Source: CAD feature listing. Evaluate the final solid. Frame: model axes, mm. A direction names the side the tool comes from. Give positions to 0.01 mm unless a question says otherwise; leave off trailing zeros. Order: outer loops, then holes, each group sorted by start corner. A loop starts at its lowest first (then second) coordinate and runs counter-clockwise, first axis right, second up.
```python
from build123d import *

# Parameters (mm, degrees)
SKETCH1_W           = 165
SKETCH1_H           = 137
BOSS_EXTRUDE1_DEPTH = 22
CUT_EXTRUDE1_DEPTH  = 165
FILLET1_R           = 3
SKETCH3_R           = 2.75
SKETCH3_R_2         = 1.45
CUT_EXTRUDE2_DEPTH  = 5
FILLET2_R           = 3
FILLET3_R           = 3


with BuildPart() as part:
    # Sketch1 → Boss-Extrude1 (new body)
    with BuildSketch(Plane(origin=(0, 0, 0), x_dir=(0, 0, -1), z_dir=(1, 0, 0))):
        Rectangle(SKETCH1_W, SKETCH1_H)
    extrude(amount=BOSS_EXTRUDE1_DEPTH)

    # Sketch2 → Cut-Extrude1 (cut)
    with BuildSketch(Plane.XY.offset(82.5)):
        Polygon((0, 48.5), (5, 48.5), (5, 53.5), (17, 53.5), (17, -53.5), (5, -53.5), (5, -43.5), (0, -43.5), align=None)
    extrude(amount=-CUT_EXTRUDE1_DEPTH, mode=Mode.SUBTRACT)

    # Fillet1
    fillet1_edges = [part.edges().sort_by_distance(p)[0] for p in [
        (22, -68.5, 0),
        (0, -43.5, 0),
        (0, 48.5, 0),
        (0, -68.5, 0),
        (0, 68.5, 0),
        (22, 68.5, 0),
    ]]
    fillet(fillet1_edges, radius=FILLET1_R)

    # Sketch3 → Cut-Extrude2 (cut)
    with BuildSketch(Plane.ZY.offset(-17)):
        with Locations(Location((0, -0.084265268, 0), (0, 0, 270))):
            Circle(SKETCH3_R)
        with Locations(Location((6.905, -0.084265268, 0), (0, 0, 270))):
            Circle(SKETCH3_R_2)
        with Locations(Location((4.882572324, -4.966837592, 0), (0, 0, 270))):
            Circle(SKETCH3_R_2)
        with Locations(Location((0, -6.989265268, 0), (0, 0, 270))):
            Circle(SKETCH3_R_2)
        with Locations(Location((-4.882572324, -4.966837592, 0), (0, 0, 270))):
            Circle(SKETCH3_R_2)
        with Locations(Location((-6.905, -0.084265268, 0), (0, 0, 270))):
            Circle(SKETCH3_R_2)
        with Locations(Location((-4.882572324, 4.798307056, 0), (0, 0, 270))):
            Circle(SKETCH3_R_2)
        with Locations(Location((0, 6.820734732, 0), (0, 0, 270))):
            Circle(SKETCH3_R_2)
        with Locations(Location((4.882572324, 4.798307056, 0), (0, 0, 270))):
            Circle(SKETCH3_R_2)
    extrude(amount=-CUT_EXTRUDE2_DEPTH, mode=Mode.SUBTRACT)

    # Fillet2
    fillet2_edges = [part.edges().sort_by_distance(p)[0] for p in [
        (4, 48.5, -82.5),
        (22, 0, -82.5),
        (0, 58.5, -82.5),
        (11, 68.5, -82.5),
        (11, -68.5, -82.5),
        (0, -56, -82.5),
        (4, -43.5, -82.5),
        (0.878679656, -44.378679656, -82.5),
        (0.878679656, 49.378679656, -82.5),
        (0.878679656, 67.621320344, -82.5),
        (21.121320344, 67.621320344, -82.5),
        (0.878679656, -67.621320344, -82.5),
        (21.121320344, -67.621320344, -82.5),
    ]]
    fillet(fillet2_edges, radius=FILLET2_R)

    # Fillet3
    fillet3_edges = [part.edges().sort_by_distance(p)[0] for p in [
        (4, 48.5, 82.5),
        (22, 0, 82.5),
        (11, -68.5, 82.5),
        (0, 58.5, 82.5),
        (4, -43.5, 82.5),
        (0, -56, 82.5),
        (11, 68.5, 82.5),
        (0.878679656, -44.378679656, 82.5),
        (0.878679656, 49.378679656, 82.5),
        (0.878679656, 67.621320344, 82.5),
        (21.121320344, 67.621320344, 82.5),
        (0.878679656, -67.621320344, 82.5),
        (21.121320344, -67.621320344, 82.5),
    ]]
    fillet(fillet3_edges, radius=FILLET3_R)


solid = part.part
```
1) Pin query (flat end, axial travel): pin 1 (1.5 mm diameter, centred on y = 49, z = 5.5, fed in from -X); pin 2 (4 mm diameter, centred on y = 4.8, z = 4.88, fed in from -X). Return the tip coordinate at first contact, or that it passes through.
Report:
pin 1: stops at x = 0.56
pin 2: stops at x = 17
2) Draft query along X for faces 3 (the flat face through (5, -49, 1)), 4 (the flat face through (17.5, -5.2, -82.5)), 5 (the flat face through (0, -56, 1)). Return one class per face: +X half, -X half, draft (parallel to the pull), parting line (faces both ways), or undercut.
Report:
face 3: undercut
face 4: draft
face 5: -X half
3) Section query C-C, the plane y = -38. Return the cut outline in (x, z), and give its area (3 significant figures).
Report:
outline: (17, -82.5) - (19, -82.5) arc R3 ccw to (22, -79.5) - (22, 79.5) arc R3 ccw to (19, 82.5) - (17, 82.5) - close
area: 821 mm2
4) Section query B-B, the plane z = 23. Return the cut outline in (x, y).
Report:
outline: (0, -65.5) arc R3 ccw to (3, -68.5) - (19, -68.5) arc R3 ccw to (22, -65.5) - (22, 65.5) arc R3 ccw to (19, 68.5) - (3, 68.5) arc R3 ccw to (0, 65.5) - (0, 51.5) arc R3 ccw to (3, 48.5) - (5, 48.5) - (5, 53.5) - (17, 53.5) - (17, -53.5) - (5, -53.5) - (5, -43.5) - (3, -43.5) arc R3 ccw to (0, -46.5) - close
5) Material intervals for L1, parallel to Y at x = 16.5, z = -62.5; L2, parallel to Y at x = 3, z = 55; L3, parallel to X at y = -46, z = 21.5, sorted ascending.
Report:
L1: y = -68.5 to -53.5, 53.5 to 68.5
L2: y = -68.5 to -43.5, 48.5 to 68.5
L3: x = 0.04 to 5, 17 to 22
6) Section query A-A, the plane x = 14.5. Return the cut outline in (y, z).
Report:
outline: (-68.5, -79.5) arc R3 ccw to (-65.5, -82.5) - (-53.5, -82.5) - (-53.5, 82.5) - (-65.5, 82.5) arc R3 ccw to (-68.5, 79.5) - close; (53.5, -82.5) - (65.5, -82.5) arc R3 ccw to (68.5, -79.5) - (68.5, 79.5) arc R3 ccw to (65.5, 82.5) - (53.5, 82.5) - close
7) Reachability of faces 1 (the flat face through (11, 68.5, 1)), 2 (the flat face through (5, 51, 1)) from +Z, -Z, +X, -X, +Y, -Y: full face, straight path, thin tool, end or side. Return the list, or none.
Report:
face 1: +Z, -Z, +X, -X, +Y
face 2: +Z, -Z
